Input: part model. Units: mm. Frame: model coordinates. A direction names the side the tool comes from. Give positions to 0.01 mm unless a question says otherwise; leave off trailing zeros. Loops run counter-clockwise (first coordinate to the right, second up) from the corner with the lowest first, then second, coordinate; pieces in that order, holes last. Notation, with made-up numbers: M 10.5,67 L 63.5,67 A18 cw 63.5,92 Z; hole C 89.5,-9.5 d6. An arc over 180 degrees is marked long. Answer as a JSON object with one key per item and string values. Group by question number.
1) Access query for faces 1 (the flat face through (47, 0, -16)), 2 (the flat face through (47, 0, 16)), 3 (the flat face through (62, 14, -6)). Directions: +Z, -Z, +X, -X, +Y, -Y. A direction counts if a zero-diameter tool reaches every point of the face in a straight line with its end or side. Return the directions, or none.
2) Draft query along X for faces 4 (the cylindrical face through (89.79, -14.18, -1.86)), 5 (the flat face through (27, -12, -4)), 6 (the flat face through (37, 0, -15)). Return one class per face: +X half, -X half, draft (parallel to the pull), parting line (faces both ways), or undercut.
3) First-contact query: P1, Ø2, axis at y = 3.5, z = 16.5, coming from the -X side; P2, Ø12, axis at x = 48, z = -2, coming from the -Y side; P3, Ø1, axis at x = 72, y = -1, coming from the -Z side; P4, Ø2, axis at x = 23, z = 0, coming from the -Y side. Flat tips, straight axial feed; report the tip coordinate or a pass-through.
4) Section query C-C on x = 10. Return loops of the section in (y, z), plus the area to 3 significant figures.
5) Section query D-D on x = 59.5. Return loops of the section in (y, z).
6) Section query B-B on y = 0. Return loops of the section in (x, z).
7) Ray query, L1, parallel to Z at x = 32.5, y = -7.5; L2, parallel to X at y = -12.5, z = 6; L3, parallel to Z at x = 11, y = -0.5. Return the intervals inside material, ascending.
8) Section query A-A on z = 0. Return loops of the section in (x, y), plus the area to 3 significant figures.
from build123d import *

# Parameters (mm, degrees)
F2_SIZE  = 1
F3_SIZE  = 1
F5_DEPTH = 12.5


with BuildPart() as f1:
    # F0 (on Front) → F1 (revolve)
    with BuildSketch(Plane.XZ):
        Polygon((0, 12), (0, 0), (94, 0), (94, 15), (90.6, 15), (90.6, 14.3), (89, 14.3), (89, 15), (62, 15), (62, 17), (27, 17), (27, 12), align=None)
    revolve(axis=Axis((47, 0, 0), (1, 0, 0)))

    # F2
    f2_edges = [f1.edges().sort_by_distance(p)[0] for p in [
        (94, 0, -15),
    ]]
    chamfer(f2_edges, length=F2_SIZE)

    # F3
    f3_edges = [f1.edges().sort_by_distance(p)[0] for p in [
        (0, 0, -12),
    ]]
    chamfer(f3_edges, length=F3_SIZE)

    # F4 (on Front) → F5 (cut, symmetric)
    with BuildSketch(Plane.XZ):
        Polygon((25.7335081697, 20.8393707871), (25.413043797, 15), (27, 15), (47, 15), (47, 20.8393707871), align=None)
        Polygon((47, -15), (27, -15), (25.413043797, -15), (25.7335081697, -20.8393707871), (47, -20.8393707871), (47, -17), align=None)
    extrude(amount=F5_DEPTH, both=True, mode=Mode.SUBTRACT)


solid = f1.part
Output:
{
 "1": {"face 1": "-Z, -X, +Y, -Y", "face 2": "+Z, -X, +Y, -Y", "face 3": "+X"},
 "2": {"face 4": "undercut", "face 5": "-X half", "face 6": "draft"},
 "3": {"P1": "stops at x = 47", "P2": "stops at y = -17", "P3": "stops at z = -14.99", "P4": "stops at y = -12"},
 "4": {"outline": "C 0,0 d24", "area": "452 mm^2"},
 "5": {"outline": "C 0,0 d34"},
 "6": {"outline": "M 0,-11 L 1,-12 L 27,-12 L 27,-15 L 47,-15 L 47,-17 L 62,-17 L 62,-15 L 89,-15 L 89,-14.3 L 90.6,-14.3 L 90.6,-15 L 93,-15 L 94,-14 L 94,14 L 93,15 L 90.6,15 L 90.6,14.3 L 89,14.3 L 89,15 L 62,15 L 62,17 L 47,17 L 47,15 L 27,15 L 27,12 L 1,12 L 0,11 Z"},
 "7": {"L1": "z = -15 to 15", "L2": "x = 27 to 94", "L3": "z = -11.99 to 11.99"},
 "8": {"outline": "M 0,-11 L 1,-12 L 27,-12 L 27,-17 L 62,-17 L 62,-15 L 89,-15 L 89,-14.3 L 90.6,-14.3 L 90.6,-15 L 93,-15 L 94,-14 L 94,14 L 93,15 L 90.6,15 L 90.6,14.3 L 89,14.3 L 89,15 L 62,15 L 62,17 L 27,17 L 27,12 L 1,12 L 0,11 Z", "area": "2,790 mm^2"}
}
